Verification items for the finished model (mm, model axes). A direction names the side the tool comes from. Round coordinates to 2 decimals unless told otherwise and drop trailing zeros. Order: outer loops, then holes, each group sorted by start corner. A loop starts at its lowest first (then second) coordinate and runs counter-clockwise, first axis right, second up. Notation, with made-up numbers: (0.25, 5.25) -> (16.25, 5.25) arc R19 cw to (16.25, 24.25) -> close; hole circle Ø4 at (-6, 69.5). An arc over 180 degrees is marked (long way). Return JSON: item names as keys, results as strings. Group by question number.
Item 1: Sectioned sample at A-A on y = -38.1. Record the cut outline in (x, z), plus the area to 3 significant figures.
Item 2: Depth check by flat-ended pin: pin 1 Ø14.5 at (x, y) = (12.7, -38.1) entering from -Z; pin 2 Ø4 at (x, y) = (11.5, -40.5) entering from -Z. Enter the tip coordinate at first touch or a pass-through.
Item 3: Scan lines: probe 1 along Y at (x, z) = (38.1, 1.75); probe 2 along X at (y, z) = (-12.7, 4.75); probe 3 along Z at (x, y) = (43.5, -11.5). Record each from-to range of solid material in increasing order. Write a range as from..to.
Item 4: Sectioned sample at B-B on x = 12.7. Record the cut outline in (y, z), plus the area to 3 significant figures.
Item 5: Draft check along Y on faces 3 (the cylindrical face through (8.02, -16.99, 3.13)), 4 (the flat face through (38, -13, 6.35)), 5 (the flat face through (25, 0, 13)), 6 (the flat face through (25, -25, 25.4)). Enter one of: pulls with the +Y half, pulls with the -Y half, needs draft (parallel to the pull), parting line crosses it, or undercut.
Item 6: Access from +Z, -Z, +X, -X, +Y, -Y to the whole of each face (thin tool, end or side, straight path). Record for faces 1 (the flat face through (25, -50.8, 13)), 2 (the flat face through (13, -38, 6.35)).
```python
from build123d import *

# Parameters (mm, degrees)
F0_W     = 50.8
F0_H     = 25.4
F1_DEPTH = 50.8
F2_R     = 6.35
F3_DEPTH = 6.35


with BuildPart() as f1:
    # F0 (on Front) → F1 (new body)
    with BuildSketch(Plane.XZ):
        with Locations((25.4, 12.7)):
            Rectangle(F0_W, F0_H)
    extrude(amount=F1_DEPTH)

    # F2 (on face) → F3 (cut)
    with BuildSketch(Plane(origin=(0, 0, 0), x_dir=(1, 0, 0), z_dir=(0, 0, -1))):
        with Locations((12.7, 38.1)):
            Circle(F2_R)
        with Locations((12.7, 12.7)):
            Circle(F2_R)
        with Locations((38.1, 12.7)):
            Circle(F2_R)
        with Locations((38.1, 38.1)):
            Circle(F2_R)
    extrude(amount=-F3_DEPTH, mode=Mode.SUBTRACT)


solid = f1.part
```
Recorded:
{
 "1": {"outline": "(0, 0) -> (6.35, 0) -> (6.35, 6.35) -> (19.05, 6.35) -> (19.05, 0) -> (31.75, 0) -> (31.75, 6.35) -> (44.45, 6.35) -> (44.45, 0) -> (50.8, 0) -> (50.8, 25.4) -> (0, 25.4) -> close", "area": "1,130 mm²"},
 "2": {"pin 1": "z = 0", "pin 2": "z = 6.35"},
 "3": {"probe 1": "-50.8..-44.45, -31.75..-19.05, -6.35..0", "probe 2": "0..6.35, 19.05..31.75, 44.45..50.8", "probe 3": "6.35..25.4"},
 "4": {"outline": "(-50.8, 0) -> (-44.45, 0) -> (-44.45, 6.35) -> (-31.75, 6.35) -> (-31.75, 0) -> (-19.05, 0) -> (-19.05, 6.35) -> (-6.35, 6.35) -> (-6.35, 0) -> (0, 0) -> (0, 25.4) -> (-50.8, 25.4) -> close", "area": "1,130 mm²"},
 "5": {"face 3": "undercut", "face 4": "undercut", "face 5": "pulls with the +Y half", "face 6": "needs draft"},
 "6": {"face 1": "+Z, -Z, +X, -X, -Y", "face 2": "-Z"}
}
